```python
from build123d import *

# Parameters (mm, degrees)
F0_R        = 6
F0_R_2      = 3.16
F1_DEPTH    = 4
F2_DEPTH    = 25
F3_S5_R     = 3.16
F3_T6_DEPTH = 10
F4_R        = 0.5


# Not quite as in the source:
# - a fillet or chamfer that OpenCascade refuses, or shapes differently, is made with other operations: its cross-section is extruded or revolved along the edge and cut away or added


with BuildPart() as f1:
    # F0 (on Top) → F1 (new body)
    with BuildSketch(Plane.XY):
        Circle(F0_R)
        Circle(F0_R_2, mode=Mode.SUBTRACT)
    extrude(amount=F1_DEPTH)

    # F0 (on Top) → F2 (join)
    with BuildSketch(Plane.XY):
        Circle(F0_R_2)
    extrude(amount=F2_DEPTH)

    # F3: chamfer of 2.85 x 3.3964977389 on 1 edges, made by hand


with BuildPart() as f3_tool2:
    # F3_s3 → F3_t4 (revolve)
    with BuildSketch(Plane.XZ):
        Polygon((6, 0.6035022611), (3.15, 4), (6, 4), align=None)
    revolve(axis=Axis((0, 0, 4), (0, 0, 1)))

    # F3_s5 → F3_t6 (cut, symmetric)
    with BuildSketch(Plane.XY.offset(2.3)):
        Circle(F3_S5_R)
    extrude(amount=F3_T6_DEPTH, both=True, mode=Mode.SUBTRACT)


with BuildPart() as f1_1:
    add(f1.part)

    # F3_t1: cut F3_tool2
    add(f3_tool2.part, mode=Mode.SUBTRACT)

    # F4
    f4_edges = [f1_1.edges().sort_by_distance(p)[0] for p in [
        (-6, 0, 0),
    ]]
    fillet(f4_edges, radius=F4_R)


solid = f1_1.part
```
Verification items for the finished model (mm, model axes). Coordinates: 2 decimals unless noted, no trailing zeros. Write each loop counter-clockwise with the first axis right and the second up, starting at its lowest first coordinate (ties: lowest second). Pieces come first, ordered by that corner, then holes. Notation, with made-up numbers: M 16.5,82 L 55.5,82 A19 cw 55.5,92 Z; hole C 22,51 d1. An arc over 180 degrees is marked long. Answer as a JSON object with one key per item and string values. Group by question number.
(1) Cross-section at D-D, the plane z = 3. Record the cut outline in (x, y), and give its area (3 significant figures).
(2) Material ranges on line 1 (X direction, y = 1.25, z = 12.25); line 2 (X direction, y = 2.5, z = 9.5); line 3 (Z direction, x = 5, y = -0.75), recorded low to high.
(3) Cross-section at C-C, the plane z = 11.5. Record the cut outline in (x, y), and give its area (3 significant figures).
(4) Cross-section at A-A, the plane y = 0. Record the cut outline in (x, z), and give its area (3 significant figures).
(5) Gauge pin test, flat ends, axial feed: pin 1 (1.5 mm diameter, centred on x = -2, z = 13, fed in from -Y); pin 2 (1 mm diameter, centred on x = -3, z = 21, fed in from +Y); pin 3 (1.5 mm diameter, centred on y = 4, z = 8, fed in from -X). Record the tip position at first contact, or that the pin passes through.
Reply:
{
 "1": {"outline": "C 0,0 d7.98", "area": "50.0 mm²"},
 "2": {"line 1": "-2.9 to 2.9", "line 2": "-1.93 to 1.93", "line 3": "0 to 1.73"},
 "3": {"outline": "C 0,0 d6.32", "area": "31.4 mm²"},
 "4": {"outline": "M -6,0.5 A0.5 ccw -5.5,0 L 5.5,0 A0.5 ccw 6,0.5 L 6,0.6 L 3.16,3.99 L 3.16,25 L -3.16,25 L -3.16,3.99 L -6,0.6 Z", "area": "171 mm²"},
 "5": {"pin 1": "y = -2.9", "pin 2": "y = 1.93", "pin 3": "through"}
}
